Read the model definition and answer for the solid it produces. Units are mm, in the model's axes. Face numbers are marked on the shaded views. Give positions to 0.01 mm unless a question says otherwise; leave off trailing zeros. Loops run counter-clockwise (first coordinate to the right, second up) from the corner with the lowest first, then second, coordinate; pieces in that order, holes last.
(1) Find section A-A, the plane y = 0. Write down the section's boundary in (x, z).
(2) Find section B-B, the plane x = 0. Write down the section's boundary in (y, z).
(3) Determine the mould class of the marked faces 1, 2 and 3 for opening direction X: pulls with the +X half, pulls with the -X half, needs draft (parallel to the pull), parting line crosses it, or undercut.
(4) Find section D-D, the plane z = 7. Write down the section's boundary in (x, y).
(5) Each of these flat-tipped pins is pushed along its axis until it touches: P1, Ø3, axis at x = 2, y = -2.5, coming from the +Z side; P2, Ø2, axis at y = 2, z = 2, coming from the +X side. Where does it stop, or does it pass through?
(6) Straight lines are drawn through the part: probe 1 along X at (y, z) = (0, 7.25); probe 2 along Z at (x, y) = (3.9, 0). For each, find the intervals that lie inside material, in ascending order.
(7) Find section C-C, the plane z = 9.25. Write down the section's boundary in (x, y), then the cut area to 3 significant figures.
Autodesk Inventor part; units mm, degrees
ref_plane "Work Plane1" through (6, 0, 0) normal (1, 0, 0) x (0, 1, 0)
ref_plane "XZ Plane" through (0, 0, 0) normal (0, 1, 0) x (-1, 0, 0)
ref_plane "XY Plane" through (0, 0, 0) normal (0, 0, 1) x (1, 0, 0)
sketch "Sketch1" plane through (0, 0, 0) normal (0, 0, 1) x (1, 0, 0)
  circle A0 centre (0, 0) radius 6
  dimension "d0" = 12
extrude "Extrusion1" add sketch "Sketch1" along normal blind 12
thread "Thread1"
ref_plane "Work Plane1" through (6, 0, 0) normal (1, 0, 0) x (0, 1, 0)
sketch "Sketch3" plane through (6, 0, 0) normal (1, 0, 0) x (0, 1, 0)
  line L0 (6, 12) -> (-6, 12)
  point P0 (0, 0)
  point P1 (0, 10)
  dimension "d13" = 2
hole "Hole2" at (6, 0, 10) direction (-1, 0, 0) diameter 3 end through all
sketch "Sketch2" plane through (0, 0, 12) normal (0, 0, 1) x (1, 0, 0)
  circle A0 centre (0, 0) radius 6
hole "Hole1" at (0, 0, 12) direction (0, 0, -1) diameter 7 depth 12
properties part number "38" material "Copper"
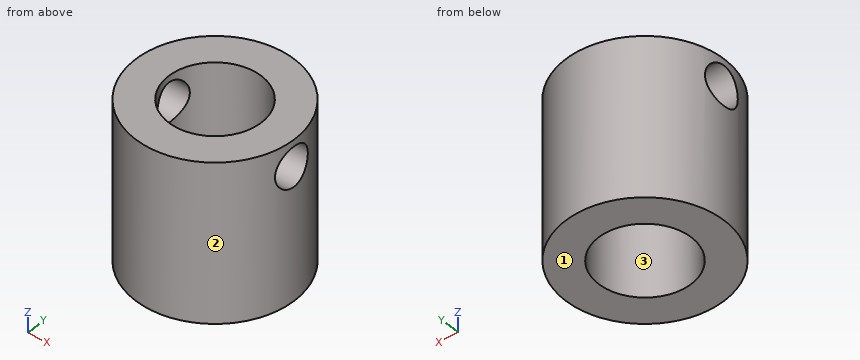
Entries:
1. outline: (-6, 0) - (-3.5, 0) - (-3.5, 8.5) - (-6, 8.5) - close; (-6, 11.5) - (-3.5, 11.5) - (-3.5, 12) - (-6, 12) - close; (3.5, 0) - (6, 0) - (6, 8.5) - (3.5, 8.5) - close; (3.5, 11.5) - (6, 11.5) - (6, 12) - (3.5, 12) - close
2. outline: (-6, 0) - (-3.5, 0) - (-3.5, 12) - (-6, 12) - close; (3.5, 0) - (6, 0) - (6, 12) - (3.5, 12) - close
3. face 1: needs draft
3. face 2: parting line crosses it
3. face 3: undercut
4. outline: circle Ø12 at (0, 0); hole circle Ø7 at (0, 0)
5. P1: stops at z = 12
5. P2: stops at x = 5.92
6. probe 1: x = -6 to -3.5, 3.5 to 6
6. probe 2: z = 0 to 8.5, 11.5 to 12
7. outline: (-5.86, -1.3) arc R6 ccw to (5.86, -1.3) - (3.25, -1.3) arc R3.5 cw to (-3.25, -1.3) - close; (-5.86, 1.3) - (-3.25, 1.3) arc R3.5 cw to (3.25, 1.3) - (5.86, 1.3) arc R6 ccw to start
7. area: 61.4 mm2
